Study the drawing (mm; zero at the part's minimum x, y, z) and answer. A direction names the side the tool comes from. Coordinates: 2 decimals unless noted, no trailing zeros. Order: outer loops, then holes, each group sorted by start corner. A loop starts at its lowest first (then second) coordinate and runs counter-clockwise, first axis right, second up. Notation, with made-up numbers: M -22.75,52 L 16.25,52 A17 ccw 16.25,81 Z; hole C 16,85 d5. An arc over 180 degrees is marked long. Use a Markdown table: item, result. Add a question column.
1) Find the intervals of material crossed by probe 1 along Y at (x, z) = (5.25, 45); probe 2 along Z at (x, y) = (3, 77); probe 3 along Y at (x, z) = (41, 29.5), in increasing order. Write a range as [from, to].
2) The mould has two halves that part along Y. Classify the marked faces 3, 4 and 5: released by +Y, released by -Y, zero draft, split by the parting line, or undercut.
3) Each of these flat-tipped pins is pushed along its axis until it touches: pin 1 Ø0.8 at (y, z) = (61.5, 20) entering from -X; pin 2 Ø8 at (x, y) = (19.5, 23.5) entering from +Z; pin 3 Ø10 at (x, z) = (38.5, 17) entering from -Y. Where does it stop, or does it pass through?
4) Find section C-C on x = 59. Write down the section's boundary in (y, z), plus the area to 3 significant figures.
5) Find section B-B on y = 66.5. Write down the section's boundary in (x, z), plus the area to 3 significant figures.
6) Find section D-D on z = 13.5. Write down the section's boundary in (x, y), plus the area to 3 significant figures.
7) Find section A-A on z = 36.5. Write down the section's boundary in (x, y).
8) For the marked faces 1 and 2, determine the directions among +Z, -Z, +X, -X, +Y, -Y from which every point of the face is accessible in a straight line to the end or side of a thin tool.
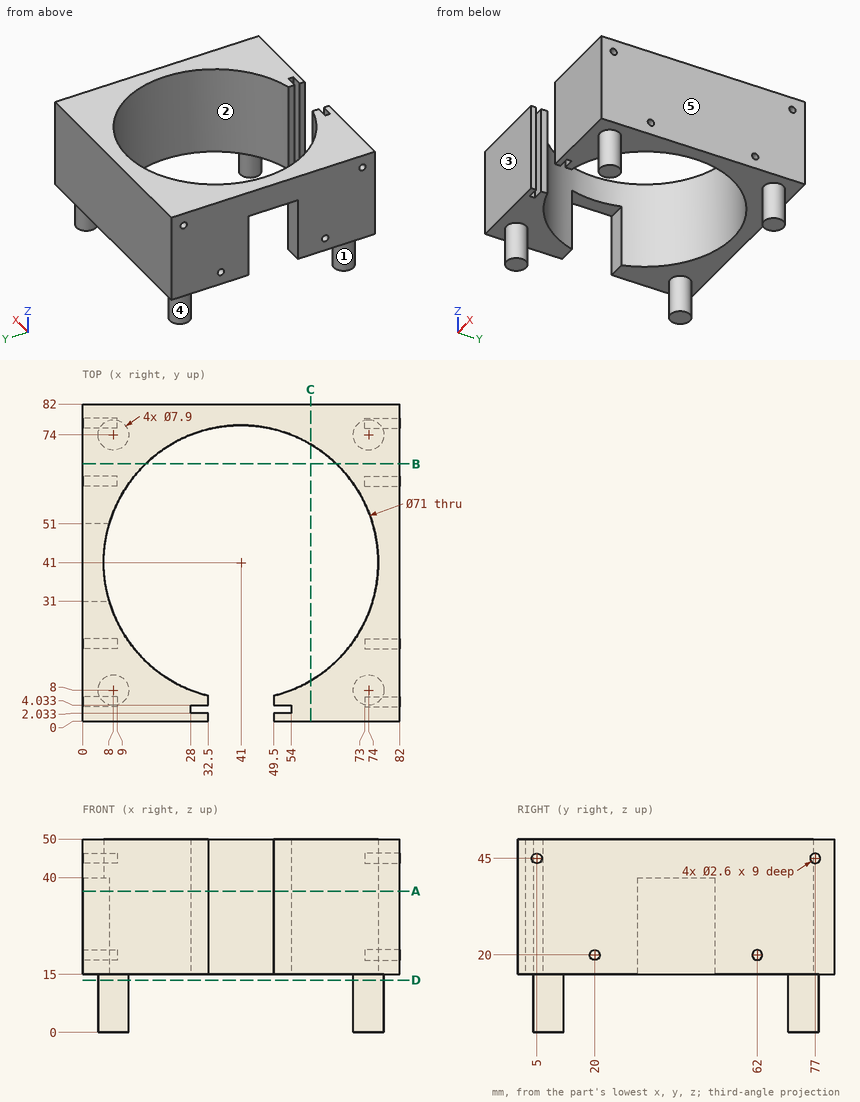
Check result:
| question | item | result |
|---|---|---|
| 1 | probe 1 | y = [0, 3.7], [6.3, 75.7], [78.3, 82] |
| 1 | probe 2 | z = [15, 43.7], [46.3, 50] |
| 1 | probe 3 | y = [76.5, 82] |
| 2 | face 3 | released by -Y |
| 2 | face 4 | undercut |
| 2 | face 5 | zero draft |
| 3 | pin 1 | stops at x = 9 |
| 3 | pin 2 | passes through |
| 3 | pin 3 | stops at y = 75.7 |
| 4 | outline | M 0,15 L 10.4,15 L 10.4,50 L 0,50 Z; M 71.6,15 L 82,15 L 82,50 L 71.6,50 Z |
| 4 | area | 728 mm2 |
| 5 | outline | M 0,15 L 16.3,15 L 16.3,50 L 0,50 Z; M 65.7,15 L 82,15 L 82,50 L 65.7,50 Z |
| 5 | area | 1,140 mm2 |
| 6 | outline | C 8,8 d7.9; C 8,74 d7.9; C 74,8 d7.9; C 74,74 d7.9 |
| 6 | area | 196 mm2 |
| 7 | outline | M 0,0 L 32.5,0 L 32.5,2.03 L 28,2.03 L 28,4.03 L 32.5,4.03 L 32.5,6.53 A35.5 cw 6.94,31 L 0,31 Z; M 0,51 L 6.94,51 A35.5 cw long 49.5,6.53 L 49.5,4.03 L 54,4.03 L 54,2.03 L 49.5,2.03 L 49.5,0 L 82,0 L 82,82 L 0,82 Z |
| 8 | face 1 | -Z |
| 8 | face 2 | +Z, -Z |
